from build123d import *

# Parameters (mm, degrees)
SKETCH1_W            = 4
SKETCH1_H            = 14
BOSS_EXTRUDE1_DEPTH  = 3
SKETCH2_R            = 1.4
BOSS_EXTRUDE2_DEPTH  = 16
SKETCH3_W            = 4
SKETCH3_H            = 1
BOSS_EXTRUDE4_DEPTH  = 6
SKETCH7_W            = 3
SKETCH7_H            = 2
BOSS_EXTRUDE5_DEPTH  = 30.95
SKETCH8_W            = 3
SKETCH8_H            = 2
BOSS_EXTRUDE6_DEPTH  = 1
SKETCH9_W            = 1
SKETCH9_H            = 2
BOSS_EXTRUDE7_DEPTH  = 3
SKETCH10_W           = 1
SKETCH10_H           = 2
BOSS_EXTRUDE8_DEPTH  = 5.92
SKETCH11_W           = 1
SKETCH11_H           = 2
BOSS_EXTRUDE9_DEPTH  = 4
SKETCH12_W           = 1
SKETCH12_H           = 3
BOSS_EXTRUDE14_DEPTH = 0.93
SKETCH13_W           = 3
SKETCH13_H           = 3
BOSS_EXTRUDE15_DEPTH = 7.1
SKETCH14_W           = 3.33402541
SKETCH14_H           = 13.860919233
CUT_EXTRUDE3_DEPTH   = 10
SKETCH15_W           = 6.20666024
SKETCH15_H           = 3.660501205
CUT_EXTRUDE4_DEPTH   = 10
SKETCH16_W           = 3
SKETCH16_H           = 9.1
BOSS_EXTRUDE16_DEPTH = 0.12
SKETCH18_W           = 3
SKETCH18_H           = 9.1
BOSS_EXTRUDE18_DEPTH = 0.41
SKETCH19_W           = 3
SKETCH19_H           = 9.1
BOSS_EXTRUDE19_DEPTH = 0.89
SKETCH20_W           = 3
SKETCH20_H           = 6
BOSS_EXTRUDE20_DEPTH = 3.77
SKETCH21_R           = 1.35
BOSS_EXTRUDE23_DEPTH = 10
BOSS_EXTRUDE24_DEPTH = 3
SKETCH24_W           = 4
SKETCH24_H           = 1
BOSS_EXTRUDE25_DEPTH = 4
SKETCH25_W           = 4
SKETCH25_H           = 7
BOSS_EXTRUDE26_DEPTH = 2
SKETCH26_W           = 6.458993184
SKETCH26_H           = 3
BOSS_EXTRUDE27_DEPTH = 7
SKETCH27_R           = 1.6
CUT_EXTRUDE5_DEPTH   = 7
SKETCH28_R           = 1.6
CUT_EXTRUDE6_DEPTH   = 7
SKETCH30_W           = 7
SKETCH30_H           = 3
BOSS_EXTRUDE29_DEPTH = 1
SKETCH31_W           = 7
SKETCH31_H           = 3
BOSS_EXTRUDE30_DEPTH = 1
SKETCH32_W           = 6
SKETCH32_H           = 7.1
BOSS_EXTRUDE31_DEPTH = 1
SKETCH33_W           = 31.638993184
SKETCH33_H           = 6
BOSS_EXTRUDE32_DEPTH = 1
SKETCH34_W           = 6
SKETCH34_H           = 14
BOSS_EXTRUDE33_DEPTH = 1


with BuildPart() as part:
    # Sketch1 → Boss-Extrude1 (new body)
    with BuildSketch(Plane.XY):
        with Locations((-1.434146341, -3.597560976)):
            Rectangle(SKETCH1_W, SKETCH1_H)
    extrude(amount=BOSS_EXTRUDE1_DEPTH)

    # Sketch2 → Boss-Extrude2 (add)
    with BuildSketch(Plane(origin=(0, 0, 0), x_dir=(-1, 0, 0), z_dir=(0, 0, -1))):
        with Locations(Location((1.434146341, 1.802439024, 0), (0, 0, 180))):
            Circle(SKETCH2_R)
    extrude(amount=BOSS_EXTRUDE2_DEPTH)

    # Sketch3 → Boss-Extrude4 (add)
    with BuildSketch(Plane.XY.offset(3)):
        with Locations((-1.434146341, -10.097560976)):
            Rectangle(SKETCH3_W, SKETCH3_H)
    extrude(amount=BOSS_EXTRUDE4_DEPTH)

    # Sketch7 → Boss-Extrude5 (add)
    with BuildSketch(Plane.ZY.offset(3.434146341)):
        with Locations((1.5, -2.497560976)):
            Rectangle(SKETCH7_W, SKETCH7_H)
    extrude(amount=BOSS_EXTRUDE5_DEPTH)

    # Sketch8 → Boss-Extrude6 (add)
    with BuildSketch(Plane.ZY.offset(34.384146341)):
        with Locations((1.5, -2.497560976)):
            Rectangle(SKETCH8_W, SKETCH8_H)
    extrude(amount=BOSS_EXTRUDE6_DEPTH)

    # Sketch9 → Boss-Extrude7 (add)
    with BuildSketch(Plane(origin=(0, 0, 0), x_dir=(-1, 0, 0), z_dir=(0, 0, -1))):
        with Locations((34.884146341, -2.497560976)):
            Rectangle(SKETCH9_W, SKETCH9_H)
    extrude(amount=BOSS_EXTRUDE7_DEPTH)

    # Sketch10 → Boss-Extrude8 (add)
    with BuildSketch(Plane(origin=(0, 0, -3), x_dir=(-1, 0, 0), z_dir=(0, 0, -1))):
        with Locations((34.884146341, -2.497560976)):
            Rectangle(SKETCH10_W, SKETCH10_H)
    extrude(amount=BOSS_EXTRUDE8_DEPTH)

    # Sketch11 → Boss-Extrude9 (add)
    with BuildSketch(Plane(origin=(0, 0, -8.92), x_dir=(-1, 0, 0), z_dir=(0, 0, -1))):
        with Locations((34.884146341, -2.497560976)):
            Rectangle(SKETCH11_W, SKETCH11_H)
    extrude(amount=BOSS_EXTRUDE9_DEPTH)

    # Sketch12 → Boss-Extrude14 (add)
    with BuildSketch(Plane.XZ.offset(3.497560976)):
        with Locations((-34.884146341, -9.28)):
            Rectangle(SKETCH12_W, SKETCH12_H)
    extrude(amount=BOSS_EXTRUDE14_DEPTH)

    # Sketch13 → Boss-Extrude15 (add)
    with BuildSketch(Plane.XZ.offset(3.497560976)):
        with Locations((-33.884146341, 1.5)):
            Rectangle(SKETCH13_W, SKETCH13_H)
    extrude(amount=BOSS_EXTRUDE15_DEPTH)

    # Sketch14 → Cut-Extrude3 (cut)
    with BuildSketch(Plane.XY.offset(3)):
        with Locations((-35.32015223, -3.66710136)):
            Rectangle(SKETCH14_W, SKETCH14_H)
    extrude(amount=-CUT_EXTRUDE3_DEPTH, mode=Mode.SUBTRACT)


with BuildPart() as cut_extrude3_piece_1:
    # of the separate pieces the step leaves, piece 1, a body of its own (cut_extrude3_pieces)
    add(part.part.solids().sort_by_distance((-3.434146341, 3.402439024, 0))[0])

    # Sketch16 → Boss-Extrude16 (add)
    with BuildSketch(Plane.ZY.offset(33.653139525)):
        with Locations((1.5, -6.047560976)):
            Rectangle(SKETCH16_W, SKETCH16_H)
    extrude(amount=BOSS_EXTRUDE16_DEPTH)

    # Sketch18 → Boss-Extrude18 (add)
    with BuildSketch(Plane.ZY.offset(33.773139525)):
        with Locations((1.5, -6.047560976)):
            Rectangle(SKETCH18_W, SKETCH18_H)
    extrude(amount=BOSS_EXTRUDE18_DEPTH)

    # Sketch19 → Boss-Extrude19 (add)
    with BuildSketch(Plane.ZY.offset(34.183139525)):
        with Locations((1.5, -6.047560976)):
            Rectangle(SKETCH19_W, SKETCH19_H)
    extrude(amount=BOSS_EXTRUDE19_DEPTH)

    # Sketch20 → Boss-Extrude20 (add)
    with BuildSketch(Plane.ZY.offset(35.073139525)):
        with Locations((1.5, -7.597560976)):
            Rectangle(SKETCH20_W, SKETCH20_H)
    extrude(amount=BOSS_EXTRUDE20_DEPTH)

    # Sketch21 → Boss-Extrude23 (add)
    with BuildSketch(Plane(origin=(0, 0, 0), x_dir=(-1, 0, 0), z_dir=(0, 0, -1))):
        with Locations(Location((36.523139525, -7.047560976, 0), (0, 0, 180))):
            Circle(SKETCH21_R)
    extrude(amount=BOSS_EXTRUDE23_DEPTH)

    # Sketch23 → Boss-Extrude24 (add)
    with BuildSketch(Plane.XY.offset(3)):
        Polygon((-38.843139525, -10.597560976), (-38.843139525, -4.597560976), (-35.073139525, -4.597560976), (-35.073139525, -1.497560976), (-3.434146341, -1.497560976), (-3.434146341, 3.402439024), (0.565853659, 3.402439024), (0.565853659, -9.597560976), (-3.434146341, -9.597560976), (-3.434146341, -3.497560976), (-32.384146341, -3.497560976), (-32.384146341, -10.597560976), align=None)
    extrude(amount=BOSS_EXTRUDE24_DEPTH)

    # Sketch24 → Boss-Extrude25 (add)
    with BuildSketch(Plane.XY.offset(9)):
        with Locations((-1.434146341, -10.097560976)):
            Rectangle(SKETCH24_W, SKETCH24_H)
    extrude(amount=BOSS_EXTRUDE25_DEPTH)

    # Sketch25 → Boss-Extrude26 (add)
    with BuildSketch(Plane(origin=(0, -9.597560976, 0), x_dir=(1, 0, 0), z_dir=(0, 1, 0))):
        with Locations((-1.434146341, -9.5)):
            Rectangle(SKETCH25_W, SKETCH25_H)
    extrude(amount=BOSS_EXTRUDE26_DEPTH)

    # Sketch26 → Boss-Extrude27 (add)
    with BuildSketch(Plane.XY.offset(6)):
        with Locations((-35.613642933, -9.097560976)):
            Rectangle(SKETCH26_W, SKETCH26_H)
    extrude(amount=BOSS_EXTRUDE27_DEPTH)

    # Sketch27 → Cut-Extrude5 (cut)
    with BuildSketch(Plane(origin=(0, -7.597560976, 0), x_dir=(1, 0, 0), z_dir=(0, 1, 0))):
        with Locations(Location((-35.613642933, -9.5, 0), (0, 0, 270))):
            Circle(SKETCH27_R)
    extrude(amount=-CUT_EXTRUDE5_DEPTH, mode=Mode.SUBTRACT)

    # Sketch28 → Cut-Extrude6 (cut)
    with BuildSketch(Plane(origin=(0, -7.597560976, 0), x_dir=(1, 0, 0), z_dir=(0, 1, 0))):
        with Locations(Location((-1.434146341, -9.5, 0), (0, 0, 270))):
            Circle(SKETCH28_R)
    extrude(amount=-CUT_EXTRUDE6_DEPTH, mode=Mode.SUBTRACT)

    # Sketch30 → Boss-Extrude29 (add)
    with BuildSketch(Plane(origin=(0.565853659, 0, 0), x_dir=(0, 0, -1), z_dir=(1, 0, 0))):
        with Locations((-9.5, -9.097560976)):
            Rectangle(SKETCH30_W, SKETCH30_H)
    extrude(amount=BOSS_EXTRUDE29_DEPTH)

    # Sketch31 → Boss-Extrude30 (add)
    with BuildSketch(Plane.ZY.offset(3.434146341)):
        with Locations((9.5, -9.097560976)):
            Rectangle(SKETCH31_W, SKETCH31_H)
    extrude(amount=BOSS_EXTRUDE30_DEPTH)

    # Sketch32 → Boss-Extrude31 (add)
    with BuildSketch(Plane.ZY.offset(3.434146341)):
        with Locations((3, -7.047560976)):
            Rectangle(SKETCH32_W, SKETCH32_H)
    extrude(amount=BOSS_EXTRUDE31_DEPTH)

    # Sketch33 → Boss-Extrude32 (add)
    with BuildSketch(Plane(origin=(0, -1.497560976, 0), x_dir=(1, 0, 0), z_dir=(0, 1, 0))):
        with Locations((-19.253642933, -3)):
            Rectangle(SKETCH33_W, SKETCH33_H)
    extrude(amount=BOSS_EXTRUDE32_DEPTH)

    # Sketch34 → Boss-Extrude33 (add)
    with BuildSketch(Plane(origin=(0.565853659, 0, 0), x_dir=(0, 0, -1), z_dir=(1, 0, 0))):
        with Locations((-3, -3.597560976)):
            Rectangle(SKETCH34_W, SKETCH34_H)
    extrude(amount=BOSS_EXTRUDE33_DEPTH)


with BuildPart() as cut_extrude3_piece_2:
    # of the separate pieces the step leaves, piece 2, a body of its own (cut_extrude3_pieces)
    add(part.part.solids().sort_by_distance((-34.384146341, -1.497560976, -7))[0])

    # Sketch15 → Cut-Extrude4 (cut)
    with BuildSketch(Plane.ZY.offset(35.384146341)):
        with Locations((-9.81666988, -3.327811578)):
            Rectangle(SKETCH15_W, SKETCH15_H)
    extrude(amount=-CUT_EXTRUDE4_DEPTH, mode=Mode.SUBTRACT)


solid = cut_extrude3_piece_1.part
Input: part model. Units: mm. Frame: model coordinates. A direction names the side the tool comes from. Round coordinates to 2 decimals unless told otherwise and drop trailing zeros. Loops run counter-clockwise (first coordinate to the right, second up) from the corner with the lowest first, then second, coordinate; pieces in that order, holes last. Notation, with made-up numbers: (26, 21) -> (34, 21) arc R25 cw to (34, 55) -> close; hole circle Ø8 at (39.5, -4.5). An arc over 180 degrees is marked (long way). Answer as a JSON object with one key per item and string values. Group by question number.
1) Section query A-A on z = 7. Output: boundary loops of the cut face in (x, y), plus the area to 3 significant figures.
2) Pin query (flat end, axial travel): pin 1 (3 mm diameter, centred on x = -28.5, y = -6, fed in from -Z); pin 2 (4 mm diameter, centred on x = -18.5, y = -1.5, fed in from -Z); pin 3 (12 mm diameter, centred on x = -34.5, z = 7.5, fed in from +Y); pin 4 (2 mm diameter, centred on y = 1, z = 3, fed in from -X). Return the tip coordinate at first contact, or that it passes through.
3) Section query D-D on z = -4.25. Output: boundary loops of the cut face in (x, y).
4) Reachability of faces 1 (the flat face through (-0.7, -7.598, 7.9)), 2 (the flat face through (-37, -4.598, 3)), 3 (the flat face through (-4.434, -8, 5)), 4 (the cylindrical face through (-37.87, -7.11, -4.93)) from +Z, -Z, +X, -X, +Y, -Y: full face, straight path, thin tool, end or side. Return the list, or none.
5) Section query B-B on x = -4. Output: boundary loops of the cut face in (y, z).
6) Section query C-C on y = 2.75. Output: boundary loops of the cut face in (x, z).
7) Ray query, L1, parallel to X at y = -9, z = 9.5; L2, parallel to X at y = -7.75, z = 3.75; L3, parallel to X at y = -3, z = 0.5. Return the intervals inside material, ascending.
8) Draft query along X for faces 5 (the flat face through (-18, -3.498, 3)), 6 (the flat face through (1.566, -5, 4)), 7 (the flat face through (-35.073, -3, 3)), 8 (the flat face through (-36, -10.598, 6)). Return one class per face: +X half, -X half, draft (parallel to the pull), parting line (faces both ways), or undercut.
Reply:
{
 "1": {"outline": "(-38.84, -10.6) -> (-32.38, -10.6) -> (-32.38, -7.6) -> (-38.84, -7.6) -> close; (-4.43, -10.6) -> (1.57, -10.6) -> (1.57, -7.6) -> (-4.43, -7.6) -> close", "area": "37.4 mm2"},
 "2": {"pin 1": "passes through", "pin 2": "stops at z = 0", "pin 3": "stops at y = -0.5", "pin 4": "stops at x = -3.43"},
 "3": {"outline": "circle Ø2.7 at (-36.52, -7.05); circle Ø2.8 at (-1.43, 1.8)"},
 "4": {"face 1": "+Z, +X, -X, +Y", "face 2": "+Z, -Z, -X, +Y", "face 3": "+Z, -Z, -Y", "face 4": "-Z"},
 "5": {"outline": "(-10.6, 0) -> (-0.5, 0) -> (-0.5, 6) -> (-7.6, 6) -> (-7.6, 13) -> (-10.6, 13) -> close"},
 "6": {"outline": "(-3.43, 0) -> (-2.46, 0) -> (-2.46, -16) -> (-0.4, -16) -> (-0.4, 0) -> (1.57, 0) -> (1.57, 6) -> (-3.43, 6) -> close"},
 "7": {"L1": "x = -38.84 to -37.21, -34.01 to -32.38, -4.43 to -3.03, 0.17 to 1.57", "L2": "x = -38.84 to -32.38, -4.43 to 1.57", "L3": "x = -35.07 to 1.57"},
 "8": {"face 5": "undercut", "face 6": "+X half", "face 7": "-X half", "face 8": "draft"}
}
